Autodesk Inventor part; units mm, degrees
ref_plane "YZ Plane" through (0, 0, 0) normal (1, 0, 0) x (0, 1, 0)
ref_plane "XZ Plane" through (0, 0, 0) normal (0, 1, 0) x (-1, 0, 0)
ref_plane "XY Plane" through (0, 0, 0) normal (0, 0, 1) x (1, 0, 0)
sketch "Эскиз1" plane through (0, 0, 0) normal (0, 0, 1) x (1, 0, 0)
  line L0 (-7.5, -27.25) -> (-4, -27.25)
  line L1 (-4, -27.25) -> (-4, -32.25)
  line L2 (-4, -32.25) -> (-1.5, -32.25)
  line L3 (-1.5, -32.25) -> (-1.5, -27.25)
  line L4 (-1.5, -27.25) -> (7.5, -27.25)
  line L5 (7.5, -4.25) -> (7.5, -27.25)
  line L6 (7.5, -4.25) -> (-1.5, -4.25)
  line L7 (-1.5, -4.25) -> (-1.5, 0.75)
  line L8 (-1.5, 0.75) -> (-4, 0.75)
  line L9 (-4, 0.75) -> (-4, -4.25)
  line L10 (-4, -4.25) -> (-7.5, -4.25)
  line L11 (-7.5, -27.25) -> (-7.5, -4.25)
  line L12 (7.5, 0) -> (6.75, 0)
  line L13 (7, 0) -> (7, -31.5)
  line L14 (-1, 0) -> (3, 0)
  arc A0 (-1, -31.5) -> (7, -31.5) centre (3, -31.5) ccw
  line L15 (-1, 0) -> (-1, -31.5)
  line L16 (7, 0) -> (7, 0.5)
  line L17 (-1, 0) -> (-1, 0.5)
  arc A1 (6.9686, 0) -> (-0.9686, 0) centre (3, 0.5) ccw
  line L18 (-1, 0) -> (-0.9686, 0)
  line L19 (6.9686, 0) -> (7, 0)
  point P0 (0, 0)
  point P1 (6.9686, 0)
  dimension "d15" = 4
  dimension "d25" = 31.5
  dimension "d26" = 0.5
  dimension "d27" = 0.5
extrude "Выдавливание1" add sketch "Эскиз1" along normal blind 3.5 contours L15 L6 L13 L4 | L4 L13 A0 L15 | L15 L14 A1 L12 L13 L6
sketch "Эскиз2" plane through (0, 0, 3.5) normal (0, 0, 1) x (1, 0, 0)
  line L0 (-7.5, -27.25) -> (-4, -27.25)
  line L1 (-4, -27.25) -> (-4, -32.25)
  line L2 (-4, -32.25) -> (-1.5, -32.25)
  line L3 (-1.5, -32.25) -> (-1.5, -27.25)
  line L4 (-1.5, -27.25) -> (7.5, -27.25)
  line L5 (7.5, -4.25) -> (7.5, -27.25)
  line L6 (7.5, -4.25) -> (-1.5, -4.25)
  line L7 (-1.5, -4.25) -> (-1.5, 0.75)
  line L8 (-1.5, 0.75) -> (-4, 0.75)
  line L9 (-4, 0.75) -> (-4, -4.25)
  line L10 (-4, -4.25) -> (-7.5, -4.25)
  line L11 (-7.5, -27.25) -> (-7.5, -4.25)
  line L12 (-1.5, -4.25) -> (7.5, -4.25)
  line L13 (7, -31.5) -> (7, 0)
  point P0 (0, 0)
sketch "Эскиз4" plane through (0, 0, 0) normal (0, 0, 1) x (1, 0, 0)
  line L0 (-0.2909, -31.25) -> (1.3546, -28.4)
  line L1 (1.3546, -28.4) -> (4.6454, -28.4)
  line L2 (4.6454, -28.4) -> (6.2909, -31.25)
  line L3 (6.2909, -31.25) -> (4.6454, -34.1)
  line L4 (4.6454, -34.1) -> (1.3546, -34.1)
  line L5 (1.3546, -34.1) -> (-0.2909, -31.25)
  arc A0 (-1, -31.5) -> (7, -31.5) centre (3, -31.5) ccw
  line L6 (-0.2909, 0.25) -> (1.3546, -2.6)
  line L7 (1.3546, -2.6) -> (4.6454, -2.6)
  line L8 (4.6454, -2.6) -> (6.2909, 0.25)
  line L9 (6.2909, 0.25) -> (4.6454, 3.1)
  line L10 (4.6454, 3.1) -> (1.3546, 3.1)
  line L11 (1.3546, 3.1) -> (-0.2909, 0.25)
  circle A1 centre (3, -31.25) radius 1.65
  circle A2 centre (3, 0.25) radius 1.65
  point P0 (0, 0)
sketch "Эскиз5" plane through (0, 0, 0) normal (0, 0, 1) x (1, 0, 0)
  circle A0 centre (3, 0.25) radius 1.65
  circle A1 centre (3, -31.25) radius 1.65
  line L0 (-1, 0) -> (-1, -31.5)
  arc A2 (-1, -31.5) -> (7, -31.5) centre (3, -31.5) ccw
  line L1 (7, -31.5) -> (7, 0)
  line L2 (6.2909, -31.25) -> (4.6454, -34.1)
  line L3 (4.6454, -34.1) -> (1.3546, -34.1)
  line L4 (1.3546, -34.1) -> (-0.2909, -31.25)
  line L5 (4.6454, -34.1) -> (1.3546, -34.1)
  line L6 (6.2909, -31.25) -> (4.6454, -34.1)
  line L7 (4.6454, -28.4) -> (6.2909, -31.25)
  line L8 (1.3546, -28.4) -> (4.6454, -28.4)
  line L9 (-0.2909, -31.25) -> (1.3546, -28.4)
  circle A3 centre (3, -31.25) radius 1.65
  line L10 (3, -15.75) -> (0.5318, -15.75)
  line L11 (7, 0) -> (6.9686, 0)
  arc A4 (6.9686, 0) -> (-0.9686, 0) centre (3, 0.5) ccw
  line L12 (-0.9686, 0) -> (-1, 0)
  point P0 (0, 0)
  dimension "d24" = 3.3
extrude "Выдавливание5" cut sketch "Эскиз5" along normal through all contours A0 | A1
sketch "Эскиз6" plane through (0, 0, 0) normal (0, 0, 1) x (1, 0, 0)
  line L0 (7.5, -4.25) -> (-1.5, -4.25)
  line L1 (-1.5, -27.25) -> (7.5, -27.25)
  line L2 (-1, 0) -> (-1, -31.5)
  line L3 (7, -31.5) -> (7, 0)
  line L4 (-1, -4.25) -> (7, -4.25)
  line L5 (7, -4.25) -> (7, -27.25)
  line L6 (7, -27.25) -> (-1, -27.25)
  line L7 (-1, -27.25) -> (-1, -4.25)
  point P0 (0, 0)
  point P1 (-1, -27.25)
extrude "Выдавливание6" cut sketch "Эскиз6" along normal blind 0.8
extrude "Выдавливание7" cut sketch "Эскиз4" along normal through all contours L0 L1 L2 L3 L4 L5 | L11 L10 L9 L8 L7 L6 | A1 | A2
sketch "Эскиз7" plane through (0, 0, 3.5) normal (0, 0, 1) x (1, 0, 0)
  line L0 (-0.2909, -31.25) -> (1.3546, -28.4)
  line L1 (1.3546, -28.4) -> (4.6454, -28.4)
  line L2 (1.3546, -34.1) -> (-0.2909, -31.25)
  line L3 (4.6454, -28.4) -> (6.2909, -31.25)
  line L4 (6.2909, -31.25) -> (4.6454, -34.1)
  line L5 (4.6454, -34.1) -> (1.3546, -34.1)
  line L6 (-1, -4.25) -> (-1, -27.25)
  line L7 (7, -27.25) -> (7, -4.25)
  line L8 (-1, -27.25) -> (-1, -15.5)
  line L9 (-1, 0) -> (-1, -31.5)
  line L10 (-1, -15.5) -> (4.3528, -15.5)
  line L11 (-0.2909, 0.25) -> (1.3546, -2.6)
  line L12 (1.3546, -2.6) -> (4.6454, -2.6)
  line L13 (1.3546, 3.1) -> (-0.2909, 0.25)
  line L14 (4.6454, -2.6) -> (6.2909, 0.25)
  line L15 (6.2909, 0.25) -> (4.6454, 3.1)
  line L16 (4.6454, 3.1) -> (1.3546, 3.1)
  point P0 (-1, 0.5)
  dimension "d31" = 11.75
extrude "Выдавливание8" cut sketch "Эскиз7" against normal blind 2.2
extrude "Выдавливание9" add sketch "Эскиз4" along normal blind 1.3 contours L0 L1 L2 L3 L4 L5 | L11 L10 L9 L8 L7 L6 | A2
sketch "Эскиз8" plane through (0, 0, 1.3) normal (0, 0, 1) x (1, 0, 0)
  circle A0 centre (3, 0.25) radius 1.65
  point P0 (0, 0)
extrude "Выдавливание10" cut sketch "Эскиз8" against normal through all
properties part number "крышка_держалка_серво_брови"
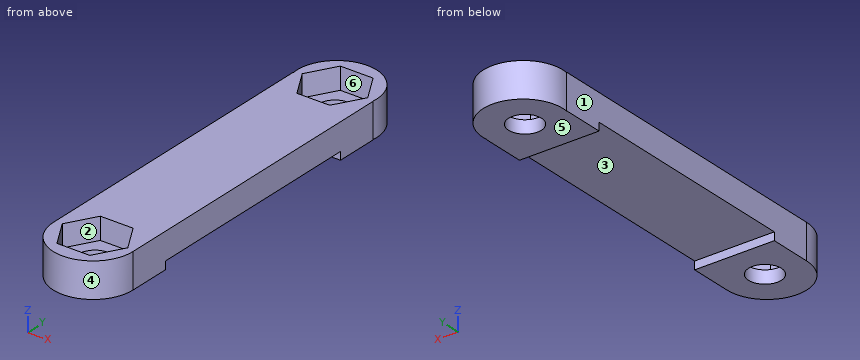
For this review, take the finished solid that the model builds, in its own axes (mm). Face numbers are marked on the shaded views. A direction names the side the tool comes from. Coordinates: 2 decimals unless noted, no trailing zeros. Loops run counter-clockwise (first coordinate to the right, second up) from the corner with the lowest first, then second, coordinate; pieces in that order, holes last.
1. For the marked faces 1, 2 and 3, list the 3-axis set-ups (+Z, -Z, +X, -X, +Y, -Y) from which the entire face can be reached by the end or side of a thin tool; tool diameter is ignored.
2. Add section B-B, the plane z = 0.35. Count the separate pieces of the cut face and the enclosed holes in it, then the cut area to 3 significant figures.
3. Add section A-A, the plane x = 3. Give the boundary of the cut face in (y, z), then the cut area to 3 significant figures.
4. Insertion check: P1, Ø0.7, axis at x = 3.5, z = 2.5, coming from the -Y side; P2, Ø2.5, axis at x = 2, y = -21, coming from the -Z side; P3, Ø2, axis at x = 6, z = 2.5, coming from the +Y side. Each pin has a flat end and moves straight along its axis. Give the tip position at first contact, or say it passes through.
5. Add section D-D, the plane x = 5.75. Give the boundary of the cut face in (y, z), then the cut area to 3 significant figures.
6. Mouldability with a two-part tool opening along Y and no side actions: class the marked faces 4, 5 and 6 as +Y half, -Y half, draft (parallel to the pull), parting line (faces both ways), or undercut.
7. For line 1 (Y direction, x = 3, z = 2.55); line 2 (Y direction, x = 3, z = 1); line 3 (Y direction, x = 2.5, z = 0.5), list the stretches that pass through material, from the lowest coordinate up.
Result:
1. face 1: +Z, -Z, -X, +Y, -Y
1. face 2: +Z
1. face 3: -Z, +X, -X
2. separate pieces: 2
2. enclosed holes: 2
2. area: 105 mm2
3. outline: (-35.5, 0) - (-32.9, 0) - (-32.9, 1.3) - (-34.1, 1.3) - (-34.1, 3.5) - (-35.5, 3.5) - close; (-29.6, 0) - (-27.25, 0) - (-27.25, 0.8) - (-4.25, 0.8) - (-4.25, 0) - (-1.4, 0) - (-1.4, 1.3) - (-2.6, 1.3) - (-2.6, 3.5) - (-28.4, 3.5) - (-28.4, 1.3) - (-29.6, 1.3) - close; (1.9, 0) - (4.5, 0) - (4.5, 3.5) - (3.1, 3.5) - (3.1, 1.3) - (1.9, 1.3) - close
3. area: 87.9 mm2
4. P1: stops at y = -35.5
4. P2: stops at z = 0.8
4. P3: stops at y = 3.96
5. outline: (-34.4, 0) - (-27.25, 0) - (-27.25, 0.8) - (-4.25, 0.8) - (-4.25, 0) - (3.4, 0) - (3.4, 3.5) - (1.19, 3.5) - (1.19, 1.3) - (-0.69, 1.3) - (-0.69, 3.5) - (-30.31, 3.5) - (-30.31, 1.3) - (-32.19, 1.3) - (-32.19, 3.5) - (-34.4, 3.5) - close
5. area: 106 mm2
6. face 4: -Y half
6. face 5: draft
6. face 6: undercut
7. line 1: y = -35.5 to -34.1, -28.4 to -2.6, 3.1 to 4.5
7. line 2: y = -35.5 to -32.9, -29.6 to -1.4, 1.9 to 4.5
7. line 3: y = -35.47 to -32.82, -29.68 to -27.25, -4.25 to -1.32, 1.82 to 4.47
